```python
from build123d import *

# Parameters (mm, degrees)
F0_W     = 31.8
F0_H     = 9.94
F0_R     = 2.4
F1_DEPTH = 9.94
F2_DEPTH = 1.67
F3_W     = 28.8
F3_H     = 6.94
F3_R     = 1.59
F4_DEPTH = 8.45


with BuildPart() as f1:
    # F0 (on Top) → F1 (new body)
    with BuildSketch(Plane.XY):
        Rectangle(F0_W, F0_H)
        with Locations((-11.82, 0)):
            Circle(F0_R, mode=Mode.SUBTRACT)
        with Locations((-3.94, 0)):
            Circle(F0_R, mode=Mode.SUBTRACT)
        with Locations((3.94, 0)):
            Circle(F0_R, mode=Mode.SUBTRACT)
        with Locations((11.82, 0)):
            Circle(F0_R, mode=Mode.SUBTRACT)
        with Locations((-11.82, 0)):
            Circle(F0_R)
        with Locations((-3.94, 0)):
            Circle(F0_R)
        with Locations((3.94, 0)):
            Circle(F0_R)
        with Locations((11.82, 0)):
            Circle(F0_R)
    extrude(amount=-F1_DEPTH)

    # F0 (on Top) → F2 (join)
    with BuildSketch(Plane.XY):
        with Locations((-11.82, 0)):
            Circle(F0_R)
        with Locations((-3.94, 0)):
            Circle(F0_R)
        with Locations((3.94, 0)):
            Circle(F0_R)
        with Locations((11.82, 0)):
            Circle(F0_R)
    extrude(amount=F2_DEPTH)

    # F3 (on face) → F4 (cut)
    with BuildSketch(Plane(origin=(0, 0, -9.94), x_dir=(1, 0, 0), z_dir=(0, 0, -1))):
        Rectangle(F3_W, F3_H)
        with Locations((-7.91, 0)):
            Circle(F3_R, mode=Mode.SUBTRACT)
        with Locations((0.17, 0)):
            Circle(F3_R, mode=Mode.SUBTRACT)
        with Locations((8.25, 0)):
            Circle(F3_R, mode=Mode.SUBTRACT)
    extrude(amount=-F4_DEPTH, mode=Mode.SUBTRACT)


solid = f1.part
```
The listing builds one solid part. Answer for the finished solid, in the listing's coordinates (mm). A direction names the side the tool comes from. Give positions to 0.01 mm unless a question says otherwise; leave off trailing zeros. Loops run counter-clockwise (first coordinate to the right, second up) from the corner with the lowest first, then second, coordinate; pieces in that order, holes last. Notation, with made-up numbers: M -15,84.5 L -1,84.5 A9 cw -1,94.5 Z; hole C 18,37.5 d5. An arc over 180 degrees is marked long. One line per item, written item: value.
1. Section A-A on z = -4.5 is taken. Determine the outline of the cut face in (x, y), plus the area to 3 significant figures.
Found:
outline: M -15.9,-4.97 L 15.9,-4.97 L 15.9,4.97 L -15.9,4.97 Z; C -7.91,0 d3.18; C 0.17,0 d3.18; C 8.25,0 d3.18; hole M -14.4,-3.47 L 14.4,-3.47 L 14.4,3.47 L -14.4,3.47 Z
area: 140 mm^2
2. For faces 1 (the face through (14, 1, 1)), 2 (the face through (-14.4, 0, -6)), 3 (the face through (-4, 0, 1.67)), determine the directions among +Z, -Z, +X, -X, +Y, -Y from which every point of the face is accessible in a straight line to the end or side of a thin tool.
Found:
face 1: +Z
face 2: -Z
face 3: +Z, +X, -X, +Y, -Y
3. Find the intervals of material crossed by probe 1 along X at (y, z) = (0, -5.75); probe 2 along Y at (x, z) = (-14, -5.75); probe 3 along X at (y, z) = (-0.75, -4.25), in increasing order.
Found:
probe 1: -15.9 to -14.4, -9.5 to -6.32, -1.42 to 1.76, 6.66 to 9.84, 14.4 to 15.9
probe 2: -4.97 to -3.47, 3.47 to 4.97
probe 3: -15.9 to -14.4, -9.31 to -6.51, -1.23 to 1.57, 6.85 to 9.65, 14.4 to 15.9
4. For a pull along Y with two mould halves and no side action, classify faces 4 (the face through (0, 3.47, -6)), 5 (the face through (0, 0, 0)), 6 (the face through (0, -4.97, -5)) as pulls with the +Y half, pulls with the -Y half, needs draft (parallel to the pull), parting line crosses it, or undercut.
Found:
face 4: undercut
face 5: needs draft
face 6: pulls with the -Y half
5. Section C-C on y = -3 is taken. Determine the outline of the cut face in (x, z), plus the area to 3 significant figures.
Found:
outline: M -15.9,-9.94 L -14.4,-9.94 L -14.4,-1.49 L 14.4,-1.49 L 14.4,-9.94 L 15.9,-9.94 L 15.9,0 L -15.9,0 Z
area: 72.7 mm^2
6. Section D-D on x = -7.91 is taken. Determine the outline of the cut face in (y, z).
Found:
outline: M -4.97,-9.94 L -3.47,-9.94 L -3.47,-1.49 L -1.59,-1.49 L -1.59,-9.94 L 1.59,-9.94 L 1.59,-1.49 L 3.47,-1.49 L 3.47,-9.94 L 4.97,-9.94 L 4.97,0 L -4.97,0 Z
7. Section B-B on x = -3.94 is taken. Determine the outline of the cut face in (y, z).
Found:
outline: M -4.97,-9.94 L -3.47,-9.94 L -3.47,-1.49 L 3.47,-1.49 L 3.47,-9.94 L 4.97,-9.94 L 4.97,0 L 2.4,0 L 2.4,1.67 L -2.4,1.67 L -2.4,0 L -4.97,0 Z
